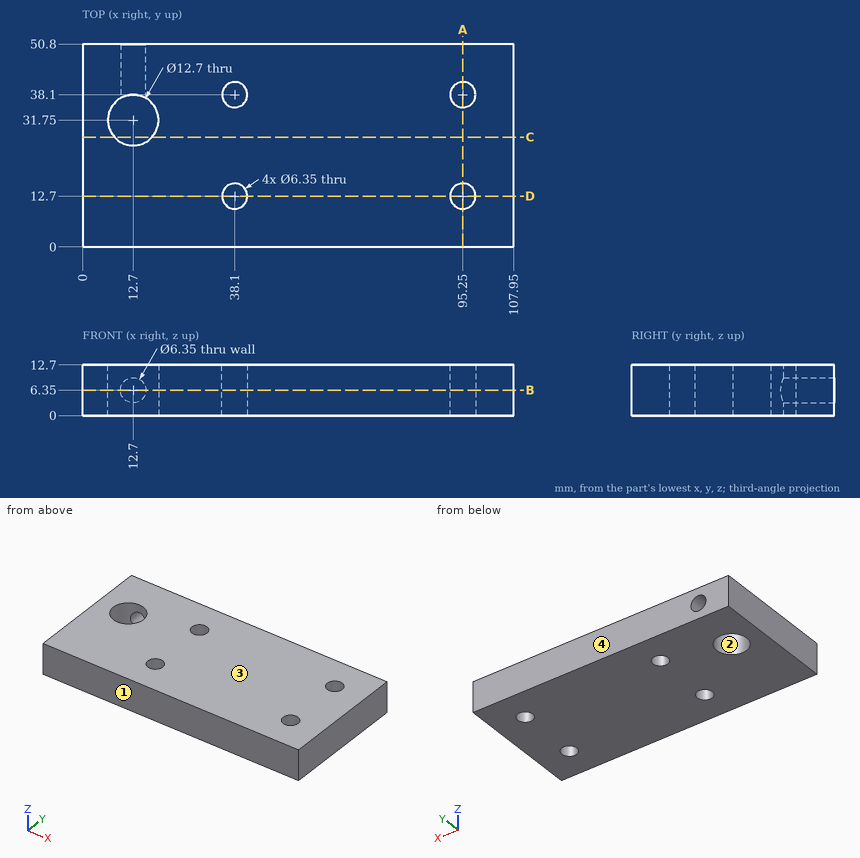
Could you check a few things on this drawing? It's one solid part, dimensions in mm from its lowest x, y, z. Round coordinates to 2 decimals unless told otherwise and drop trailing zeros. Order: outer loops, then holes, each group sorted by start corner. A loop starts at its lowest first (then second) coordinate and runs counter-clockwise, first axis right, second up.
Q1. Imagine slicing it at C-C, the plane y = 27.5. List the corners of the cut face in (x, z) for me.
Geometry says:
outline: (0, 0) - (7.98, 0) - (7.98, 12.7) - (0, 12.7) - close; (17.42, 0) - (107.95, 0) - (107.95, 12.7) - (17.42, 12.7) - close
Q2. Imagine slicing it at D-D, the plane y = 12.7. List the corners of the cut face in (x, z) for me (3 decimals), then the cut area to 3 significant figures.
Geometry says:
outline: (0, 0) - (34.925, 0) - (34.925, 12.7) - (0, 12.7) - close; (41.275, 0) - (92.075, 0) - (92.075, 12.7) - (41.275, 12.7) - close; (98.425, 0) - (107.95, 0) - (107.95, 12.7) - (98.425, 12.7) - close
area: 1,210 mm2
Q3. Imagine slicing it at A-A, the plane x = 95.25. List the corners of the cut face in (y, z) for me (3 decimals).
Geometry says:
outline: (0, 0) - (9.525, 0) - (9.525, 12.7) - (0, 12.7) - close; (15.875, 0) - (34.925, 0) - (34.925, 12.7) - (15.875, 12.7) - close; (41.275, 0) - (50.8, 0) - (50.8, 12.7) - (41.275, 12.7) - close
Q4. Imagine slicing it at B-B, the plane z = 6.35. List the corners of the cut face in (x, y) for me (3 decimals).
Geometry says:
outline: (0, 0) - (107.95, 0) - (107.95, 50.8) - (15.875, 50.8) - (15.875, 37.249) arc R6.35 cw (long way) to (9.525, 37.249) - (9.525, 50.8) - (0, 50.8) - close; hole circle Ø6.35 at (38.1, 12.7); hole circle Ø6.35 at (38.1, 38.1); hole circle Ø6.35 at (95.25, 12.7); hole circle Ø6.35 at (95.25, 38.1)
Q5. Thinking about a two-plate mould opening in Y: for the marked faces 1, 2, 3 and 4, which applies, released by +Y, released by -Y, zero draft, split by the parting line, or undercut?
Geometry says:
face 1: released by -Y
face 2: undercut
face 3: zero draft
face 4: released by +Y
Q6. Please list where these lines run through material, in increasing order: probe 1 along Y at (x, z) = (95, 12.25); probe 2 along X at (y, z) = (35.5, 10.25); probe 3 along Z at (x, y) = (12.7, 44) (3 decimals).
Geometry says:
probe 1: y = 0 to 9.53, 15.87 to 34.93, 41.27 to 50.8
probe 2: x = 0 to 7.58, 17.82 to 36.28, 39.92 to 93.43, 97.07 to 107.95
probe 3: z = 0 to 3.175, 9.525 to 12.7
